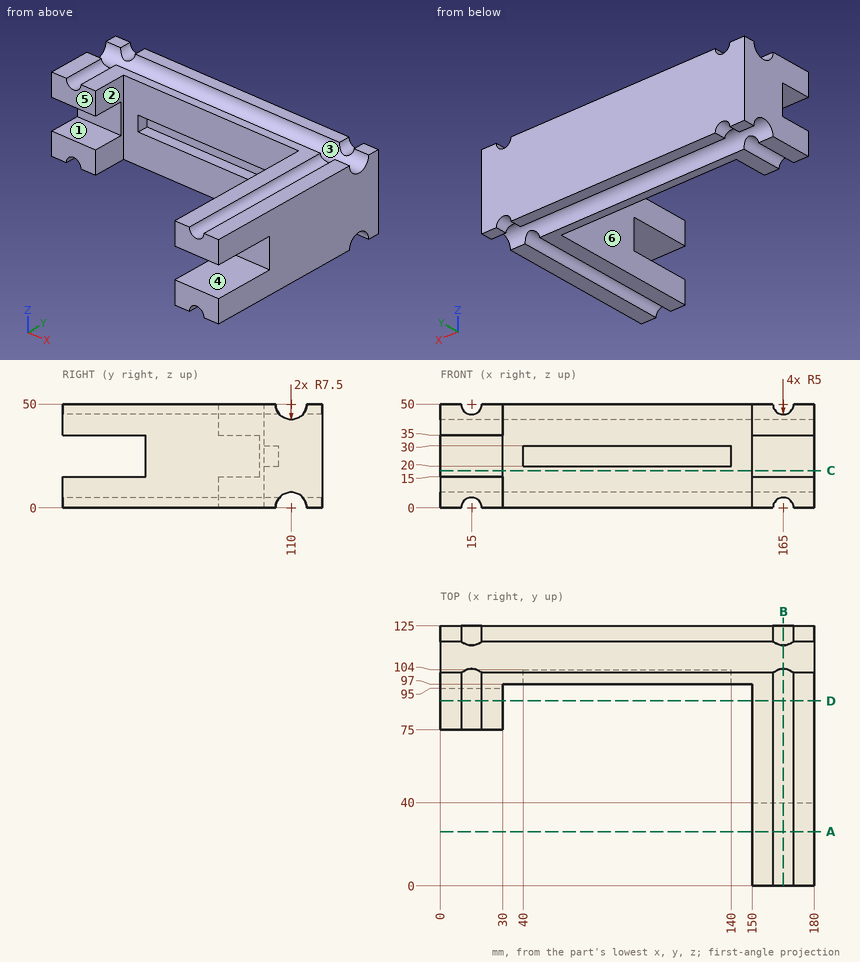
Study the drawing (mm; zero at the part's minimum x, y, z) and answer. A direction names the side the tool comes from. Coordinates: 2 decimals unless noted, no trailing zeros. Loops run counter-clockwise (first coordinate to the right, second up) from the corner with the lowest first, then second, coordinate; pieces in that order, holes last. Notation, with made-up numbers: M 88,-22.5 L 130,-22.5 A28 cw 130,6.5 Z; hole C 13,14 d5. An arc over 180 degrees is marked long. Answer in a Markdown table with one row per item. Add a question column.
1. Find section B-B, the plane x = 165. Write down the section's boundary in (y, z).
2. Find section D-D, the plane y = 89. Write down the section's boundary in (x, z), then the cut area to 3 significant figures.
3. Find section A-A, the plane y = 26. Write down the section's boundary in (x, z), then the cut area to 3 significant figures.
4. A tool of negligible diameter and unlimited length cuts with its end or side. For the marked faces 4, 5 and 6, from which of +Z, -Z, +X, -X, +Y, -Y can it reach the whole face along a straight path? Write none if from no direction.
5. The mould has two halves that part along Z. Classify the marked faces 1, 2 and 3: pulls with the +Z half, pulls with the -Z half, needs draft (parallel to the pull), parting line crosses it, or undercut.
6. Find section C-C, the plane z = 18. Write down the section's boundary in (x, y).
7. Consider L1, parallel to X at y = 96, z = 28; L2, parallel to Y at x = 163.5, z = 45; L3, parallel to X at y = 98.5, z = 21. Determine where each line is inside the solid, lowest interval first.
8. Flat-ended cylindrical pins translate along their axes: P1, Ø2, axis at x = 72, z = 10, coming from the -Y side; P2, Ø10, axis at x = 161.5, z = 26, coming from the -Y side; P3, Ø7.5, axis at x = 20.5, z = 11, coming from the -Y side; P4, Ø6, axis at x = 17.5, y = 86, coming from the +Z side. Find the tip coordinate at first contact, or state that the pin passes through.
Reported:
| question | item | result |
|---|---|---|
| 1 | outline | M 0,5 L 104.41,5 A7.5 cw 115.59,5 L 125,5 L 125,45 L 115.59,45 A7.5 cw 104.41,45 L 0,45 L 0,35 L 40,35 L 40,15 L 0,15 Z |
| 2 | outline | M 0,0 L 10,0 A5 cw 20,0 L 30,0 L 30,15 L 0,15 Z; M 0,35 L 30,35 L 30,50 L 20,50 A5 cw 10,50 L 0,50 Z; M 150,0 L 160,0 A5 cw 170,0 L 180,0 L 180,50 L 170,50 A5 cw 160,50 L 150,50 Z |
| 2 | area | 2,240 mm^2 |
| 3 | outline | M 150,0 L 160,0 A5 cw 170,0 L 180,0 L 180,15 L 150,15 Z; M 150,35 L 180,35 L 180,50 L 170,50 A5 cw 160,50 L 150,50 Z |
| 3 | area | 821 mm^2 |
| 4 | face 4 | +X, -X, -Y |
| 4 | face 5 | +Z, -Z, -X, -Y |
| 4 | face 6 | +Z, -Z, -Y |
| 5 | face 1 | undercut |
| 5 | face 2 | needs draft |
| 5 | face 3 | pulls with the +Z half |
| 6 | outline | M 0,95 L 30,95 L 30,97 L 150,97 L 150,40 L 180,40 L 180,125 L 0,125 Z |
| 7 | L1 | x = 0 to 30, 150 to 180 |
| 7 | L2 | y = 0 to 104.41, 115.59 to 125 |
| 7 | L3 | x = 0 to 40, 140 to 180 |
| 8 | P1 | stops at y = 97 |
| 8 | P2 | stops at y = 40 |
| 8 | P3 | stops at y = 75 |
| 8 | P4 | stops at z = 50 |
